Read the model definition and answer for the solid it produces. Units are mm, in the model's axes. Coordinates: 2 decimals unless noted, no trailing zeros. Loops run counter-clockwise (first coordinate to the right, second up) from the corner with the lowest first, then second, coordinate; pieces in that order, holes last. Notation, with made-up numbers: (2, 65.5) - (14, 65.5) arc R23 ccw to (14, 93.5) - close; hole circle Ø11 at (8.25, 12.5). An arc over 180 degrees is marked (long way). Use CSV: the item, a comma, the result in double quotes.
```python
from build123d import *

# Parameters (mm, degrees)
F0_R     = 10.668
F0_R_2   = 7.8994
F1_DEPTH = 203.2
F2_R     = 10.668
F2_R_2   = 7.8994
F3_DEPTH = 25.4


with BuildPart() as f1:
    # F0 (on Top) → F1 (new body)
    with BuildSketch(Plane.XY):
        Circle(F0_R)
        Circle(F0_R_2, mode=Mode.SUBTRACT)
    extrude(amount=F1_DEPTH)

    # F2 (on Front) → F3 (cut)
    with BuildSketch(Plane.XZ):
        with Locations((0.5100271213, 102.0716684638)):
            Circle(F2_R)
        with Locations((0.5100271213, 102.0716684638)):
            Circle(F2_R_2, mode=Mode.SUBTRACT)
        with Locations((0.5100271213, 102.0716684638)):
            Circle(F2_R_2)
    extrude(amount=-F3_DEPTH, mode=Mode.SUBTRACT)


solid = f1.part
```
Q1. The part is cut by section B-B on x = -4.5. Determine the outline of the cut face in (y, z).
Reported:
outline,"(-9.67, 0) - (-6.49, 0) - (-6.49, 203.2) - (-9.67, 203.2) - close; (6.49, 0) - (9.67, 0) - (9.67, 92.65) - (6.49, 92.65) - close; (6.49, 111.49) - (9.67, 111.49) - (9.67, 203.2) - (6.49, 203.2) - close"
Q2. The part is cut by section C-C on z = 80. Determine the outline of the cut face in (x, y).
Reported:
outline,"circle Ø21.34 at (0, 0); hole circle Ø15.8 at (0, 0)"
Q3. Find the intervals of material crossed by probe 1 along X at (y, z) = (0.75, 57); probe 2 along Y at (x, z) = (2.5, 165); probe 3 along Y at (x, z) = (3, 84), in increasing order. Write a range as [from, to].
Reported:
probe 1,"x = [-10.64, -7.86], [7.86, 10.64]"
probe 2,"y = [-10.37, -7.49], [7.49, 10.37]"
probe 3,"y = [-10.24, -7.31], [7.31, 10.24]"
Q4. For a pull along Z with two mould halves and no side action, classify faces 1 (the face through (-7, -4, 203.2)), 2 (the face through (-7, -4, 0)), 3 (the face through (-8.357, 5.273, 96.141)) as +Z half, -Z half, draft (parallel to the pull), parting line (faces both ways), or undercut.
Reported:
face 1,"+Z half"
face 2,"-Z half"
face 3,"undercut"
Q5. Given P1, Ø8, axis at x = 0.5, z = 105, coming from the +Y side; P2, Ø3, axis at y = -2.5, z = 99.5, coming from the +X side; P3, Ø1.5, axis at x = 2.5, z = 45.5, coming from the +Y side, each flat-ended and moving along its own axis, determine where each tip first touches the part or whether it passes through.
Reported:
P1,"stops at y = -6.49"
P2,"stops at x = 10.62"
P3,"stops at y = 10.52"
Q6. The part is cut by section A-A on y = 2. Determine the outline of the cut face in (x, z), and give its area (3 significant figures).
Reported:
outline,"(-10.48, 0) - (-7.64, 0) - (-7.64, 95.19) arc R10.67 cw to (-7.64, 108.95) - (-7.64, 203.2) - (-10.48, 203.2) - close; (7.64, 0) - (10.48, 0) - (10.48, 98.27) arc R10.67 cw to (7.64, 94.14) - close; (7.64, 110.01) arc R10.67 cw to (10.48, 105.87) - (10.48, 203.2) - (7.64, 203.2) - close"
area,"1,090 mm²"
